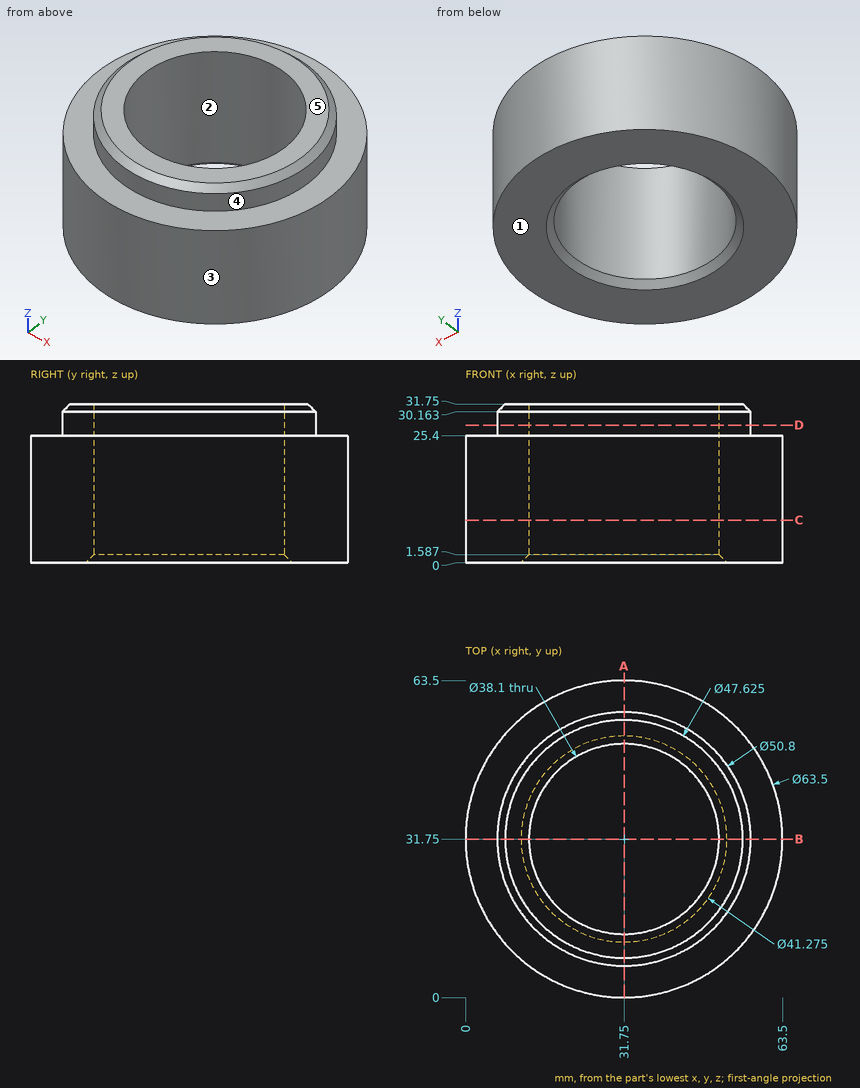
The drawing under review shows one solid part. Ordinate dimensions are in mm from its lowest x, y, z. A direction names the side the tool comes from. Give positions to 0.01 mm unless a question says otherwise; leave off trailing zeros. Loops run counter-clockwise (first coordinate to the right, second up) from the corner with the lowest first, then second, coordinate; pieces in that order, holes last. Notation, with made-up numbers: M -27.5,-2 L 30.5,-2 A8 ccw 30.5,6 Z; hole C 71.25,18.5 d5. An arc over 180 degrees is marked long. One line per item, written item: value. Start each with the question number.
Q1. Clearance check with flat-ended pins moving along their axes: pin 1 Ø12 at (x, z) = (24, 26.5) entering from +Y; pin 2 Ø12 at (y, z) = (51, 12.5) entering from +X; pin 3 Ø8 at (x, z) = (52.5, 25.5) entering from +Y. State where each tip first meets the part, or that it passes through.
Q2. For L1, parallel to Y at x = 31.75, z = 14.5; L2, parallel to Y at x = 14.5, z = 20.5 (1 decimal); L3, parallel to X at y = 28.5, z = 15.5, list the stretches that pass through material, from the lowest coordinate up.
Q3. Draft analysis for pull direction X (two halves, no side actions). For the marked faces 1, 2 and 3, state which applies: released by +X, released by -X, zero draft, split by the parting line, or undercut.
Q4. Add section A-A (x = 31.75). Give the boundary of the cut face in (y, z), and give its area (3 significant figures).
Q5. Add section C-C (z = 8.5). Give the boundary of the cut face in (x, y), and give its area (3 significant figures).
Q6. Add section D-D (z = 27.5). Give the boundary of the cut face in (x, y).
Q7. Machinability: for the marked faces 4 and 5, which of the approach directions +Z, -Z, +X, -X, +Y, -Y give a long, thin tool a straight path to every point of the face, cutting with its end or side? Answer none if there is none.
Reply:
1. pin 1: y = 63.45
1. pin 2: x = 60.6
1. pin 3: y = 58.72
2. L1: 0 to 12.7, 50.8 to 63.5
2. L2: 5.1 to 23.7, 39.8 to 58.4
2. L3: 0.17 to 12.98, 50.52 to 63.33
3. face 1: zero draft
3. face 2: undercut
3. face 3: split by the parting line
4. outline: M 0,0 L 11.11,0 L 12.7,1.59 L 12.7,31.75 L 7.94,31.75 L 6.35,30.16 L 6.35,25.4 L 0,25.4 Z; M 50.8,1.59 L 52.39,0 L 63.5,0 L 63.5,25.4 L 57.15,25.4 L 57.15,30.16 L 55.56,31.75 L 50.8,31.75 Z
4. area: 721 mm²
5. outline: C 31.75,31.75 d63.5; hole C 31.75,31.75 d38.1
5. area: 2,030 mm²
6. outline: C 31.75,31.75 d50.8; hole C 31.75,31.75 d38.1
7. face 4: +Z
7. face 5: +Z, +X, -X, +Y, -Y
